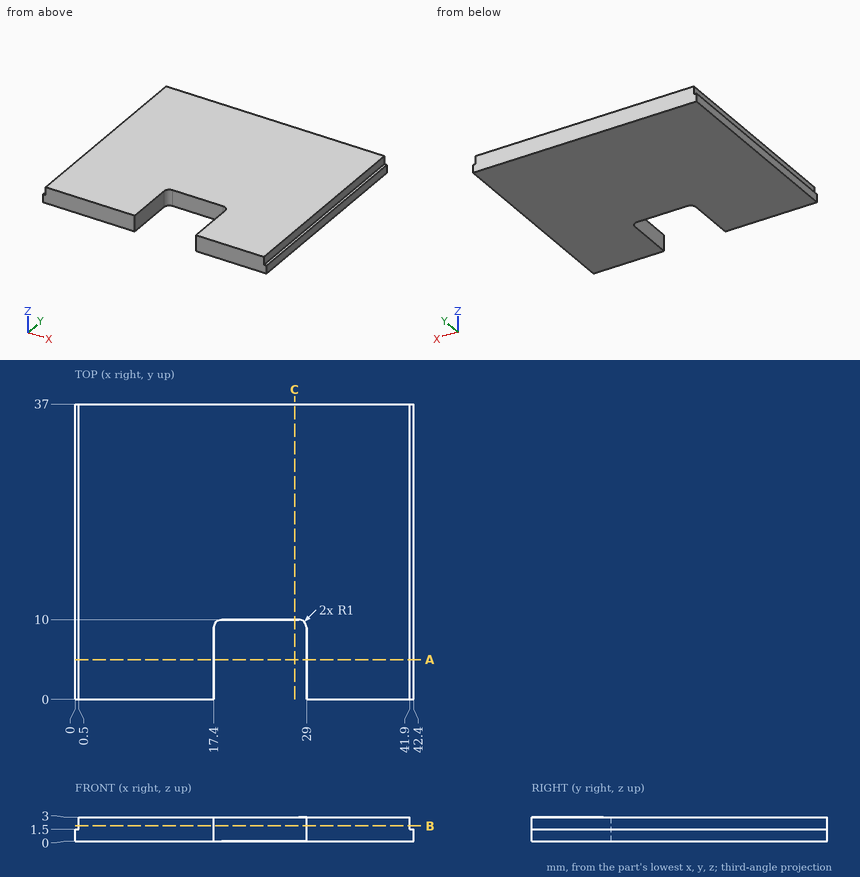
Part print with two shaded views. Sizes in mm from the minimum x, y, z corner. Round coordinates to 2 decimals unless told otherwise and drop trailing zeros. Order: outer loops, then holes, each group sorted by start corner. A loop starts at its lowest first (then second) coordinate and runs counter-clockwise, first axis right, second up. Notation, with made-up numbers: (-40, 38) - (18, 38) arc R23 ccw to (18, 73) - close; hole circle Ø6 at (75, 69). An arc over 180 degrees is marked (long way). Return JSON: item names as keys, results as strings.
(1) Cut at C-C (x = 27.5). Give the cut face in (y, z), then the cut area to 3 significant figures.
Answer key:
{"outline": "(10, 0) - (37, 0) - (37, 3) - (10, 3) - close", "area": "81.0 mm^2"}
(2) Wall check: probe 1 along X at (y, z) = (3, 1.45); probe 2 along X at (y, z) = (21.5, 2.05); probe 3 along Y at (x, z) = (28, 2.4). Give the ranges that are in metal, low to high. Write a range as from..to.
Answer key:
{"probe 1": "x = 0..17.4, 29..42.4", "probe 2": "x = 0.5..41.9", "probe 3": "y = 10..37"}
(3) Cut at B-B (z = 1.95). Give the cut face in (x, y), then the cut area to 3 significant figures.
Answer key:
{"outline": "(0.5, 0) - (17.4, 0) - (17.4, 9) arc R1 cw to (18.4, 10) - (28, 10) arc R1 cw to (29, 9) - (29, 0) - (41.9, 0) - (41.9, 37) - (0.5, 37) - close", "area": "1,420 mm^2"}
(4) Pin check, flat tips, straight feed: pin 1 Ø0.8 at (y, z) = (18.5, 2) entering from +X; pin 2 Ø0.9 at (x, z) = (21.5, 1) entering from -Y; pin 3 Ø0.8 at (y, z) = (26.5, 2) entering from -X. Stop position of each tip, or through.
Answer key:
{"pin 1": "stops at x = 41.9", "pin 2": "stops at y = 10", "pin 3": "stops at x = 0.5"}
(5) Cut at A-A (y = 5). Give the cut face in (x, z), then the cut area to 3 significant figures.
Answer key:
{"outline": "(0, 0) - (17.4, 0) - (17.4, 3) - (0.5, 3) - (0.5, 1.5) - (0, 1.5) - close; (29, 0) - (42.4, 0) - (42.4, 1.5) - (41.9, 1.5) - (41.9, 3) - (29, 3) - close", "area": "90.9 mm^2"}
